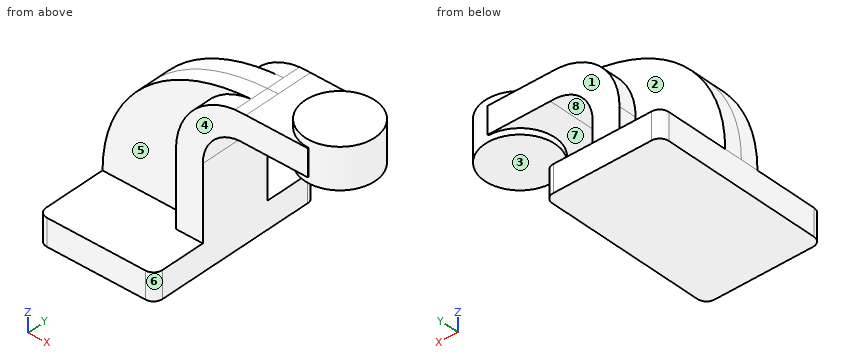
```python
from build123d import *

# Parameters (mm, degrees)
F1_DEPTH = 2.5
F0_W     = 1.0246116972
F0_H     = 0.75
F2_DEPTH = 1
F3_DEPTH = 0.5
F5_R     = 0.25
F6_SCALE = 10


with BuildPart() as f1:
    # F0 (on Front) → F1 (new body, symmetric)
    with BuildSketch(Plane.XZ):
        Polygon((-1.625, 0.375), (-1.625, -0.375), (1.625, -0.375), (1.625, 0.375), (0.875, 0.375), align=None)
    extrude(amount=F1_DEPTH, both=True)

    # F0 (on Front) → F2 (join, symmetric)
    with BuildSketch(Plane.XZ):
        with BuildLine():
            Line((0.875, 0.375), (1.625, 0.375))
            Line((1.625, 0.375), (1.625, 2.435))
            ThreePointArc((1.625, 2.435), (1.9763518814, 3.2395897205), (2.8053269877, 3.5287489089))
            Line((2.8053269877, 3.5287489089), (3.5307152905, 3.5287489089))
            Line((3.5307152905, 3.5287489089), (3.5307152905, 4.2787489089))
            Line((3.5307152905, 4.2787489089), (2.8301783535, 4.2787489089))
            add(Edge.make_bspline(
                [(2.5259841505, 4.2715011565), (2.6257724531, 4.2763068408), (2.7271772665, 4.2787489089), (2.8301783535, 4.2787489089)],
                knots=[5.7079224482, 5.7079224482, 5.7079224482, 5.7079224482, 5.9235014734, 5.9235014734, 5.9235014734, 5.9235014734], degree=3))
            ThreePointArc((2.5259841505, 4.2715011565), (1.3484222124, 3.6697555591), (0.875, 2.435))
            Line((0.875, 2.435), (0.875, 0.375))
        make_face()
        with Locations((4.0430211391, 3.9037489089)):
            Rectangle(F0_W, F0_H)
    extrude(amount=F2_DEPTH, both=True)

    # F0 (on Front) → F3 (join, symmetric)
    with BuildSketch(Plane.XZ):
        with BuildLine():
            add(Edge.make_bspline(
                [(-1.625, 0.375), (-1.625, 2.3600286686), (-0.1161276805, 4.1442602386), (2.5259841505, 4.2715011565)],
                knots=[0, 0, 0, 0, 5.7079224482, 5.7079224482, 5.7079224482, 5.7079224482], degree=3))
            Line((-1.625, 0.375), (0.875, 0.375))
            Line((0.875, 0.375), (0.875, 2.435))
            ThreePointArc((0.875, 2.435), (1.3484222124, 3.6697555591), (2.5259841505, 4.2715011565))
        make_face()
    extrude(amount=F3_DEPTH, both=True)

    # F0 (on Front) → F4 (revolve)
    with BuildSketch(Plane.XZ):
        Polygon((4.5553269877, 4.4876907729), (4.5553269877, 4.2787489089), (4.5553269877, 3.5287489089), (4.5553269877, 3.3626907729), (5.5307152905, 3.3626907729), (5.5307152905, 4.4876907729), align=None)
    revolve(axis=Axis((4.5553269877, 0, 3.9251907729), (0, 0, 1)))

    # F5
    f5_edges = [f1.edges().sort_by_distance(p)[0] for p in [
        (1.625, -2.5, 0),
        (-1.625, -2.5, 0),
        (1.625, 2.5, 0),
        (-1.625, 2.5, 0),
    ]]
    fillet(f5_edges, radius=F5_R)


with BuildPart() as f1_1:
    # F6: moved
    add(f1.part.scale(F6_SCALE))


solid = f1_1.part
```
Part model, mm, in its own coordinate system. Face numbers are marked on the shaded views. A direction names the side the tool comes from. Coordinates: 2 decimals unless noted, no trailing zeros. Write each loop counter-clockwise with the first axis right and the second up, starting at its lowest first coordinate (ties: lowest second). Pieces come first, ordered by that corner, then holes.
Item 1: Which spindle directions (+Z, -Z, +X, -X, +Y, -Y) get a long thin tool onto all of the face, cutting with end or side? Do the marked faces 1, 2, 3 and 4. Say none if no direction does.
Item 2: Slice it at A-A (y = -13.5). Write the cut outline in (x, z).
Item 3: Pin check, flat tips, straight feed: pin 1 (4 mm diameter, centred on y = 8.5, z = 16.5, fed in from -X); pin 2 (18.5 mm diameter, centred on x = 20, z = 31.5, fed in from +Y); pin 3 (4 mm diameter, centred on y = -8.5, z = 10.5, fed in from -X). Stop position of each tip, or through.
Item 4: Mould opens along X. For the marked faces 5, 6, 7 and 8 say: released by +X, released by -X, zero draft, split by the parting line, or undercut.
Item 5: Slice it at B-B (x = 40). Write the cut outline in (y, z), and give its area (3 significant figures).
Item 6: Probe line 1 (Z direction, x = 42, y = 5); line 2 (Z direction, x = 8.5, y = -8); line 3 (Y direction, x = 14.5, z = 34.5). List the from-to ranges inside material, lowest first.
Results found:
1. face 1: +Z, +X, -X, +Y
1. face 2: +Z, -X, +Y
1. face 3: -Z, +X, +Y, -Y
1. face 4: +Z, +X, -X, -Y
2. outline: (-16.25, -3.75) - (16.25, -3.75) - (16.25, 3.75) - (-16.25, 3.75) - close
3. pin 1: stops at x = 8.75
3. pin 2: stops at y = 10
3. pin 3: stops at x = 8.75
4. face 5: zero draft
4. face 6: released by +X
4. face 7: undercut
4. face 8: undercut
5. outline: (-10, 35.29) - (-8.02, 35.29) - (-8.02, 33.63) - (8.02, 33.63) - (8.02, 35.29) - (10, 35.29) - (10, 42.79) - (8.02, 42.79) - (8.02, 44.88) - (-8.02, 44.88) - (-8.02, 42.79) - (-10, 42.79) - close
5. area: 210 mm2
6. line 1: z = 33.63 to 44.88
6. line 2: z = -3.75 to 3.75
6. line 3: y = -10 to 10
